Answer from the drawing. Dimensions are ordinates in mm from the lowest x, y and z of the part. A direction names the side the tool comes from. Give positions to 0.01 mm unless a question says otherwise; leave off trailing zeros. Loops run counter-clockwise (first coordinate to the right, second up) from the corner with the lowest first, then second, coordinate; pieces in that order, holes last. Notation, with made-up numbers: (-20.5, 74) - (6.5, 74) arc R28 cw to (6.5, 106) - close; hole circle Ø4 at (83.25, -29.75). An arc over 180 degrees is marked (long way). One line per item, written item: value.
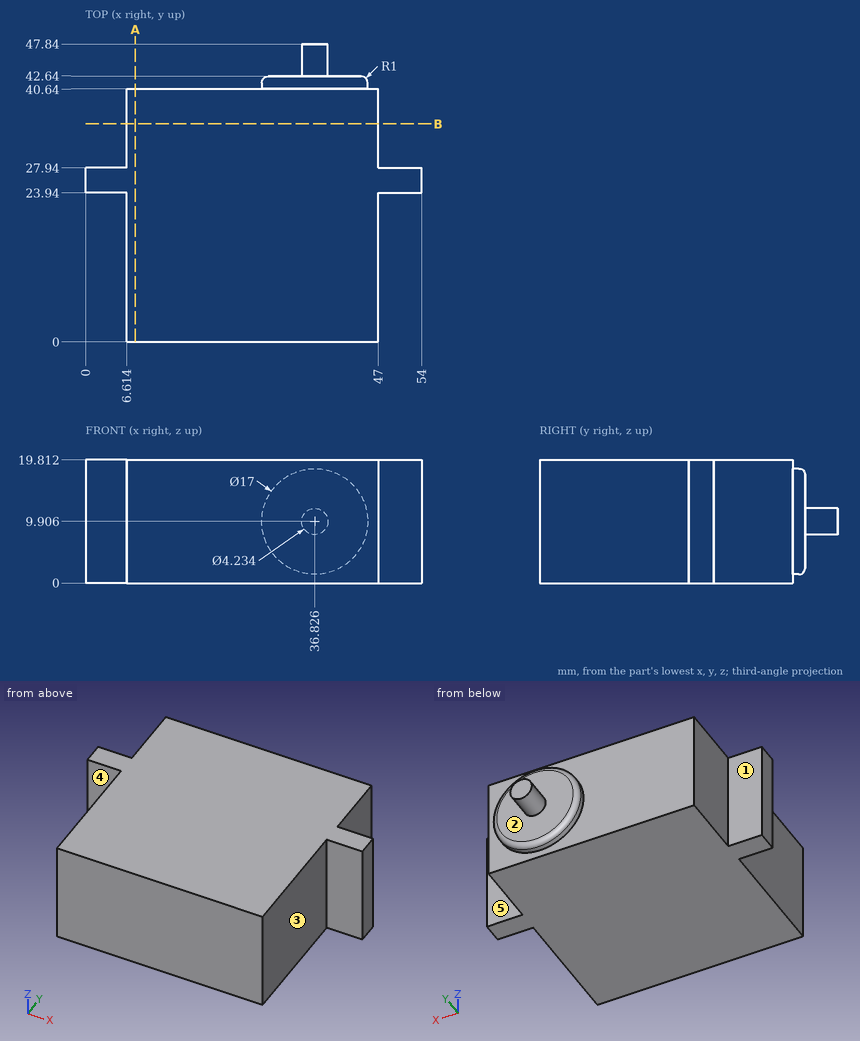
1. Flat-ended cylindrical pins translate along their axes: pin 1 Ø8 at (x, z) = (34.5, 3) entering from -Y; pin 2 Ø3.5 at (x, z) = (50.5, 15) entering from +Y; pin 3 Ø1 at (y, z) = (10.5, 11.5) entering from +X; pin 4 Ø6 at (y, z) = (16.5, 6) entering from -X. Find the tip coordinate at first contact, or state that the pin passes through.
Output:
pin 1: stops at y = 0
pin 2: stops at y = 27.94
pin 3: stops at x = 47
pin 4: stops at x = 6.61
2. Section A-A (x = 8) is taken. Write down the section's boundary in (y, z).
Output:
outline: (0, 0) - (40.64, 0) - (40.64, 19.81) - (0, 19.81) - close
3. Find the intervals of material crossed by line 1 along X through (y, z) = (7, 11.25); line 2 along Y through (x, z) = (40, 13.25); line 3 along Y through (x, z) = (5.5, 5), in increasing order.
Output:
line 1: x = 6.61 to 47
line 2: y = 0 to 42.64
line 3: y = 23.94 to 27.94
4. For the marked faces 1, 2, 3, 4 and 5, determine the directions among +Z, -Z, +X, -X, +Y, -Y from which every point of the face is accessible in a straight line to the end or side of a thin tool.
Output:
face 1: +Z, -Z, -X, +Y
face 2: +Y
face 3: +Z, -Z, +X, -Y
face 4: +Z, -Z, -X, -Y
face 5: +Z, -Z, +X, +Y
5. Section B-B (y = 35) is taken. Write down the section's boundary in (x, z).
Output:
outline: (6.61, 0) - (47, 0) - (47, 19.81) - (6.61, 19.81) - close
